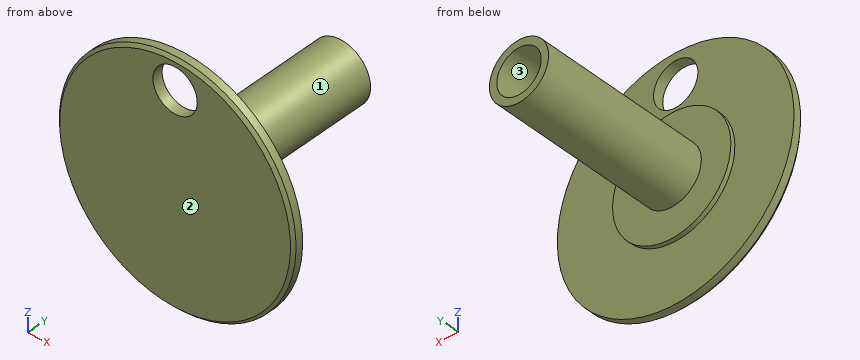
from build123d import *

# Parameters (mm, degrees)
SKETCH1_R           = 8
BOSS_EXTRUDE1_DEPTH = 0.7
SKETCH2_R           = 4
BOSS_EXTRUDE2_DEPTH = 0.3
SKETCH3_R           = 2
BOSS_EXTRUDE3_DEPTH = 11.6
SKETCH4_R           = 1.5
CUT_EXTRUDE1_DEPTH  = 8.5
SKETCH5_R           = 1.5
CUT_EXTRUDE2_DEPTH  = 17.933989489
CHAMFER1_SIZE       = 0.2


with BuildPart() as part:
    # Sketch1 → Boss-Extrude1 (new body)
    with BuildSketch(Plane(origin=(0, 0, 0), x_dir=(1, 0, 0), z_dir=(0, 1, 0))):
        with Locations(Location((0, 0, 0), (0, 0, 270))):
            Circle(SKETCH1_R)
    extrude(amount=BOSS_EXTRUDE1_DEPTH)

    # Sketch2 → Boss-Extrude2 (add)
    with BuildSketch(Plane(origin=(0, 0.7, 0), x_dir=(1, 0, 0), z_dir=(0, 1, 0))):
        with Locations(Location((0, 0, 0), (0, 0, 270))):
            Circle(SKETCH2_R)
    extrude(amount=BOSS_EXTRUDE2_DEPTH)

    # Sketch3 → Boss-Extrude3 (add)
    with BuildSketch(Plane(origin=(0, 1, 0), x_dir=(1, 0, 0), z_dir=(0, 1, 0))):
        with Locations(Location((0, 0, 0), (0, 0, 270))):
            Circle(SKETCH3_R)
    extrude(amount=BOSS_EXTRUDE3_DEPTH)

    # Sketch4 → Cut-Extrude1 (cut)
    with BuildSketch(Plane(origin=(0, 12.6, 0), x_dir=(1, 0, 0), z_dir=(0, 1, 0))):
        with Locations(Location((0, 0, 0), (0, 0, 270))):
            Circle(SKETCH4_R)
    extrude(amount=-CUT_EXTRUDE1_DEPTH, mode=Mode.SUBTRACT)

    # Sketch5 → Cut-Extrude2 (cut, through all)
    with BuildSketch(Plane.XZ):
        with Locations(Location((0, 6, 0), (0, 0, 270))):
            Circle(SKETCH5_R)
    extrude(amount=-CUT_EXTRUDE2_DEPTH, mode=Mode.SUBTRACT)

    # Chamfer1
    chamfer1_edges = [part.edges().sort_by_distance(p)[0] for p in [
        (0, 0, -8),
    ]]
    chamfer(chamfer1_edges, length=CHAMFER1_SIZE)


solid = part.part
Geometry check sheet. Reference: the model listing, model coordinates, mm. Face numbers are marked on the shaded views. Give positions to 0.01 mm unless a question says otherwise; leave off trailing zeros. Order: outer loops, then holes, each group sorted by start corner. A loop starts at its lowest first (then second) coordinate and runs counter-clockwise, first axis right, second up. Notation, with made-up numbers: M 54,20 L 73,20 A23 ccw 73,48 Z; hole C 24,87 d9. An arc over 180 degrees is marked long. Use a Markdown table: item, result.
Item 1: Section check C-C (y = 7.5). Record the cut outline in (x, z).
Answers follow:
| item | result |
|---|---|
| outline | C 0,0 d4; hole C 0,0 d3 |
Item 2: Material ranges on line 1 along X through (y, z) = (8.5, 0); line 2 along Y through (x, z) = (-4.75, 0.25); line 3 along Y through (x, z) = (-1, 2), recorded low to high.
Answers follow:
| item | result |
|---|---|
| line 1 | x = -2 to -1.5, 1.5 to 2 |
| line 2 | y = 0 to 0.7 |
| line 3 | y = 0 to 1 |
Item 3: Draft check along Z on the marked faces 1, 2 and 3. Enter one of: +Z half, -Z half, draft (parallel to the pull), parting line (faces both ways), or undercut.
Answers follow:
| item | result |
|---|---|
| face 1 | parting line |
| face 2 | draft |
| face 3 | undercut |
Item 4: Depth check by flat-ended pin: P1, Ø0.9, axis at x = -0.5, z = 0.5, coming from the +Y side; P2, Ø2, axis at x = 6, z = 1.5, coming from the +Y side; P3, Ø5, axis at x = 4, z = -4.5, coming from the +Y side. Enter the tip coordinate at first touch or a pass-through.
Answers follow:
| item | result |
|---|---|
| P1 | stops at y = 4.1 |
| P2 | stops at y = 0.7 |
| P3 | stops at y = 1 |
Item 5: Section check A-A (x = 0). Record the cut outline in (y, z).
Answers follow:
| item | result |
|---|---|
| outline | M 0,-7.8 L 0.2,-8 L 0.7,-8 L 0.7,-4 L 1,-4 L 1,-2 L 12.6,-2 L 12.6,-1.5 L 4.1,-1.5 L 4.1,1.5 L 12.6,1.5 L 12.6,2 L 1,2 L 1,4 L 0.7,4 L 0.7,4.5 L 0,4.5 Z; M 0,7.5 L 0.7,7.5 L 0.7,8 L 0.2,8 L 0,7.8 Z |
Item 6: Section check B-B (z = 0). Record the cut outline in (x, y), and give its area (3 significant figures).
Answers follow:
| item | result |
|---|---|
| outline | M -8,0.2 L -7.8,0 L 7.8,0 L 8,0.2 L 8,0.7 L 4,0.7 L 4,1 L 2,1 L 2,12.6 L 1.5,12.6 L 1.5,4.1 L -1.5,4.1 L -1.5,12.6 L -2,12.6 L -2,1 L -4,1 L -4,0.7 L -8,0.7 Z |
| area | 34.5 mm2 |
Item 7: Section check D-D (y = 2). Record the cut outline in (x, z), and give its area (3 significant figures).
Answers follow:
| item | result |
|---|---|
| outline | C 0,0 d4 |
| area | 12.6 mm2 |
